Autodesk Inventor part; units mm, degrees
ref_plane "YZ Plane" through (0, 0, 0) normal (1, 0, 0) x (0, 1, 0)
ref_plane "XZ Plane" through (0, 0, 0) normal (0, 1, 0) x (-1, 0, 0)
ref_plane "XY Plane" through (0, 0, 0) normal (0, 0, 1) x (1, 0, 0)
sketch "Sketch1" plane through (0, 0, 0) normal (0, 1, 0) x (-1, 0, 0)
  line L0 (0, 0) -> (63.5, 0)
  line L1 (63.5, 0) -> (63.5, 127)
  line L2 (63.5, 127) -> (0, 127)
  line L3 (0, 127) -> (0, 0)
  dimension "d0" = 63.5
  dimension "d1" = 127
extrude "Extrusion1" add sketch "Sketch1" along normal blind 12.7
sketch "Sketch2" plane through (0, 12.7, 0) normal (0, 1, 0) x (1, 0, 0)
  line L0 (0, 0) -> (0, -25.4)
  line L1 (0, -127) -> (0, 0)
  line L2 (0, 0) -> (-63.5, 0)
  line L3 (0, 0) -> (-63.5, 0)
  line L4 (-63.5, 0) -> (-63.5, -25.4)
  line L5 (-63.5, 0) -> (-63.5, -127)
  line L6 (-63.5, -25.4) -> (0, -25.4)
  dimension "d4" = 25.4
extrude "Extrusion2" add sketch "Sketch2" along normal blind 25.4
properties part number "hook"
Check sheet for the modelled part. Datum: model origin and axes. Units: mm. A direction names the side the tool comes from. Round coordinates to 2 decimals unless told otherwise and drop trailing zeros. Order: outer loops, then holes, each group sorted by start corner. A loop starts at its lowest first (then second) coordinate and runs counter-clockwise, first axis right, second up.
Q1. Set-up check for faces 1 (the face through (-63.5, 10, 48)), 2 (the face through (-31, 12.7, 77)): record each of +Z, -Z, +X, -X, +Y, -Y from which the full face is reachable in a straight line by a thin tool's end or side.
Filled sheet:
face 1: +Z, -Z, -X, +Y, -Y
face 2: +Z, +X, -X, +Y
Q2. Depth check by flat-ended pin: P1, Ø10, axis at x = -29.5, y = 24, coming from the +Z side; P2, Ø12, axis at x = -51, z = 82.5, coming from the +Y side. Enter the tip coordinate at first touch or a pass-through.
Filled sheet:
P1: stops at z = 25.4
P2: stops at y = 12.7
Q3. Cross-section at C-C, the plane y = 17.5. Enter the section's corners in (x, z).
Filled sheet:
outline: (-63.5, 0) - (0, 0) - (0, 25.4) - (-63.5, 25.4) - close
Q4. Cross-section at B-B, the plane z = 110.5. Enter the section's corners in (x, y).
Filled sheet:
outline: (-63.5, 0) - (0, 0) - (0, 12.7) - (-63.5, 12.7) - close
Q5. Scan lines: L1, parallel to Z at x = -29, y = 19.5; L2, parallel to Y at x = -38.5, z = 91.5. Record each from-to range of solid material in increasing order.
Filled sheet:
L1: z = 0 to 25.4
L2: y = 0 to 12.7
Q6. Cross-section at A-A, the plane x = -54.5. Enter the section's corners in (y, z), plus the area to 3 significant figures.
Filled sheet:
outline: (0, 0) - (38.1, 0) - (38.1, 25.4) - (12.7, 25.4) - (12.7, 127) - (0, 127) - close
area: 2,260 mm2
